Verification items for the finished model (mm, model axes). A direction names the side the tool comes from. Give positions to 0.01 mm unless a question says otherwise; leave off trailing zeros. Loops run counter-clockwise (first coordinate to the right, second up) from the corner with the lowest first, then second, coordinate; pieces in that order, holes last. Notation, with made-up numbers: M -2.5,29.25 L 53.5,29.25 A27 cw 53.5,52.25 Z; hole C 43,46.25 d4. An arc over 180 degrees is marked long. Use CSV: the item, a comma, the result in double quotes.
from build123d import *

# Parameters (mm, degrees)
SKETCH1_R                       = 4
SKETCH1_R_2                     = 87.5
BOSS_EXTRUDE1_DEPTH             = 17
CBORE_FOR_M10_SHCS1_D           = 11
CBORE_FOR_M10_SHCS1_CBORE_D     = 18
CBORE_FOR_M10_SHCS1_CBORE_DEPTH = 10
F_3_8_16_TAPPED_HOLE3_D         = 7.9375


with BuildPart() as part:
    # Sketch1 → Boss-Extrude1 (new body)
    with BuildSketch(Plane.XY):
        with BuildLine():
            Line((-131.19643785, -89.124723518), (66.8670709, -152.795612062))
            ThreePointArc((66.8670709, -152.795612062), (77.933659306, -153.140329428), (87.494178001, -147.556003928))
            Line((87.494178001, -147.556003928), (138.994178001, -93.615245818))
            ThreePointArc((138.994178001, -93.615245818), (142.158380517, -89.25120713), (144.044882633, -84.201640712))
            Line((144.044882633, -84.201640712), (174.718661169, 51.290400995))
            ThreePointArc((174.718661169, 51.290400995), (173.689671163, 63.379486111), (165.873431227, 72.659097776))
            Line((165.873431227, 72.659097776), (80.089309433, 126.829422905))
            ThreePointArc((80.089309433, 126.829422905), (-77.284768492, 128.557631275), (-149.578321741, -11.239469072))
            Line((-149.578321741, -11.239469072), (-145.046651368, -71.548336401))
            ThreePointArc((-145.046651368, -71.548336401), (-140.803414929, -82.449846894), (-131.19643785, -89.124723518))
        make_face()
        with Locations((-125.063508749, -70.046782494)):
            Circle(SKETCH1_R, mode=Mode.SUBTRACT)
        with Locations((73.000000001, -133.717671038)):
            Circle(SKETCH1_R, mode=Mode.SUBTRACT)
        with Locations((124.500000001, -79.776912929)):
            Circle(SKETCH1_R, mode=Mode.SUBTRACT)
        with Locations((155.173778537, 55.715128778)):
            Circle(SKETCH1_R, mode=Mode.SUBTRACT)
        with Locations((-32, 129.301071167)):
            Circle(SKETCH1_R, mode=Mode.SUBTRACT)
        Circle(SKETCH1_R_2, mode=Mode.SUBTRACT)
        with Locations((-124.734461308, 44.232368469)):
            Circle(SKETCH1_R, mode=Mode.SUBTRACT)
    extrude(amount=BOSS_EXTRUDE1_DEPTH)

    # CBORE for M10 SHCS1 (through all)
    with Locations(Plane(origin=(-124.734461308, 44.232368469, 17), x_dir=(1, 0, 0), z_dir=(0, 0, 1))):
        with Locations((0, 0), (92.734461308, 85.068702698), (279.908239845, 11.482760309), (249.234461309, -124.009281398), (197.734461309, -177.950039507), (-0.329047441, -114.279150963)):
            CounterBoreHole(CBORE_FOR_M10_SHCS1_D / 2, CBORE_FOR_M10_SHCS1_CBORE_D / 2, CBORE_FOR_M10_SHCS1_CBORE_DEPTH)

    # 3/8-16 Tapped Hole3 (through all)
    with Locations(Plane(origin=(-48.728615608, 94.900708221, 17), x_dir=(1, 0, 0), z_dir=(0, 0, 1))):
        with Locations((0, 0), (143.629323829, -46.172092613), (97.457231216, -189.801416442), (-46.172092613, -143.629323829)):
            Hole(F_3_8_16_TAPPED_HOLE3_D / 2)


solid = part.part
(1) Scan lines: L1, parallel to X at y = -68.5, z = 12; L2, parallel to X at y = 60, z = 5.5; L3, parallel to X at y = 51.5, z = 11.75. Record each from-to range of solid material in increasing order. Write a range as from..to.
Calculated:
L1,"x = -145.28..-133.93, -116.2..-54.44, 54.44..147.6"
L2,"x = -137.48..-63.69, 63.69..151.73, 158.62..174.75"
L3,"x = -140.88..-130.04, -119.43..-70.74, 70.74..92.06, 97.74..147.22, 163.13..174.76"
(2) Depth check by flat-ended pin: pin 1 Ø7 at (x, y) = (48.73, -94.9) entering from +Z; pin 2 Ø10 at (x, z) = (18, 14.5) entering from -Y; pin 3 Ø6 at (x, z) = (78, 6.5) entering from -Y; pin 4 Ø9 at (x, y) = (-29, 131.5) entering from +Z. Enter the tip coordinate at first touch or a pass-through.
Calculated:
pin 1,"passes through"
pin 2,"stops at y = -138.69"
pin 3,"stops at y = -153.66"
pin 4,"stops at z = 7"
(3) Section check A-A on y = 0. Record the cut outline in (x, z).
Calculated:
outline,"M -150,0 L -87.5,0 L -87.5,17 L -150,17 Z; M 87.5,0 L 163.11,0 L 163.11,17 L 87.5,17 Z"
(4) Section check D-D on z = 2.75. Count the separate pieces of the cut face and the enclosed holes in it, plus the area to 3 significant figures.
Calculated:
separate pieces,"1"
enclosed holes,"11"
area,"49,100 mm²"
(5) Section check B-B on x = 0. Record the cut outline in (y, z), plus the area to 3 significant figures.
Calculated:
outline,"M -131.3,0 L -87.5,0 L -87.5,17 L -131.3,17 Z; M 87.5,0 L 150,0 L 150,17 L 87.5,17 Z"
area,"1,810 mm²"
(6) Tool access check on faces 4 (the flat face through (159, 60, 7)), 5 (the cylindrical face through (-64.49, 59.14, 8.38)). Record the directions out of +Z, -Z, +X, -X, +Y, -Y that give a thin tool (end or side, any length) a straight path to the whole face; none if there is none.
Calculated:
face 4,"+Z"
face 5,"+Z, -Z"
(7) Mould release check, pull along Y, two halves, no side actions. Record for faces 1 (the flat face through (159.17, -17.4, 8.38)), 2 (the flat face through (-36, 125, 7)), 3 (the flat face through (83, 34, 17)): released by +Y, released by -Y, zero draft, split by the parting line, or undercut.
Calculated:
face 1,"released by -Y"
face 2,"undercut"
face 3,"zero draft"
(8) Section check C-C on x = 73. Record the cut outline in (y, z).
Calculated:
outline,"M -153.76,0 L -139.22,0 L -139.22,7 L -142.72,7 L -142.72,17 L -153.76,17 Z; M -128.22,0 L -48.24,0 L -48.24,17 L -124.72,17 L -124.72,7 L -128.22,7 Z; M 48.24,0 L 131.04,0 L 131.04,17 L 48.24,17 Z"
